Geometry: see drawing. Coordinates: mm, zero at the bounding-box minimum. A direction names the side the tool comes from. Round coordinates to 2 decimals unless told otherwise and drop trailing zeros. Order: outer loops, then holes, each group sorted by start corner. A loop starts at its lowest first (then second) coordinate and runs counter-clockwise, first axis right, second up. Notation, with made-up numbers: (-40, -7) - (-16, -7) arc R19 cw to (-16, 1) - close; hole circle Ø11 at (34, 36). An arc over 180 degrees is marked (long way). Put each result on its own line as item: value. Start each with the question number.
1) Line query: probe 1 along Y at (x, z) = (66.25, 0.65); probe 2 along Z at (x, y) = (16, 28.5); probe 3 along X at (y, z) = (20, 6.5). Output: solid intervals per line, ascending. Write a range as [from, to].
2) Section A-A on y = 28. Output: boundary loops of the cut face in (x, z), then the cut area to 3 significant figures.
3) Mould query, pull axis Y, two halves, no side actions, for the marked faces 1 and 2. Classes: +Y half, -Y half, draft (parallel to the pull), parting line (faces both ways), or undercut.
4) Section C-C on y = 11. Output: boundary loops of the cut face in (x, z).
5) Section D-D on z = 4.5. Output: boundary loops of the cut face in (x, y).
6) Contact query for flat-ended pins moving along their axis: P1, Ø5, axis at x = 57.5, y = 9.5, coming from the +Z side; P2, Ø5, axis at x = 66, y = 11, coming from the +Z side; P3, Ø0.8, axis at x = 65.5, z = 2.5, coming from the +Y side; P4, Ø4, axis at x = 10.5, z = 2.5, coming from the +Y side. Output: stop coordinate, or through.
7) Access query for the marked faces 3 and 4. Directions: +Z, -Z, +X, -X, +Y, -Y. A direction counts if a zero-diameter tool reaches every point of the face in a straight line with its end or side. Return the directions, or none.
8) Section B-B on x = 66.25. Output: boundary loops of the cut face in (y, z), then the cut area to 3 significant figures.
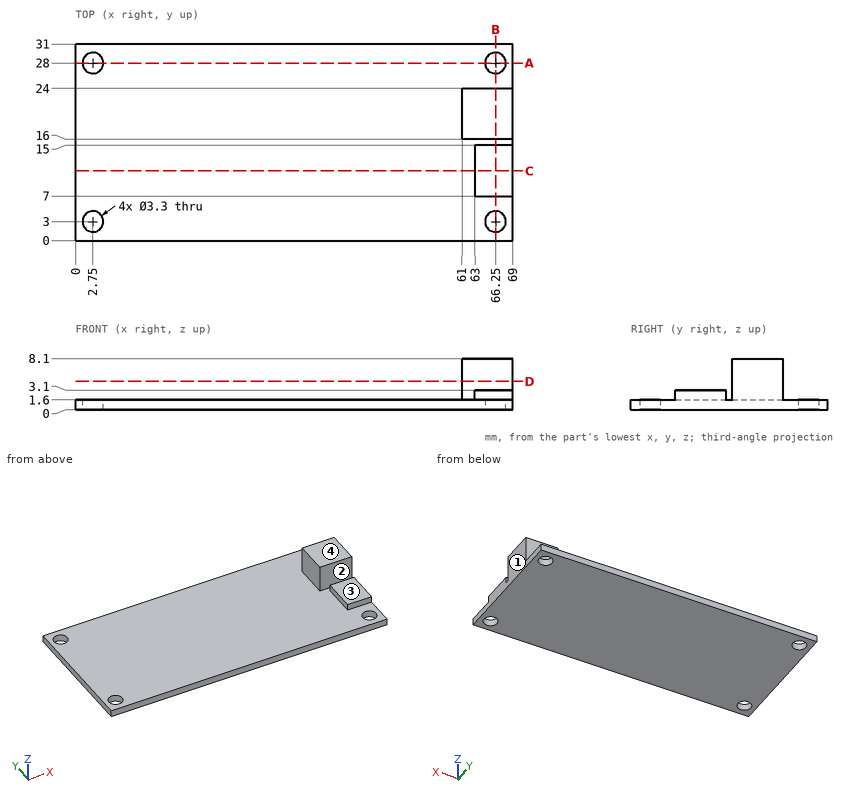
Answer sheet:
1. probe 1: [0, 1.35], [4.65, 26.35], [29.65, 31]
1. probe 2: [0, 1.6]
1. probe 3: [61, 69]
2. outline: (0, 0) - (1.1, 0) - (1.1, 1.6) - (0, 1.6) - close; (4.4, 0) - (64.6, 0) - (64.6, 1.6) - (4.4, 1.6) - close; (67.9, 0) - (69, 0) - (69, 1.6) - (67.9, 1.6) - close
2. area: 99.8 mm^2
3. face 1: draft
3. face 2: undercut
4. outline: (0, 0) - (69, 0) - (69, 3.1) - (63, 3.1) - (63, 1.6) - (0, 1.6) - close
5. outline: (61, 16) - (69, 16) - (69, 24) - (61, 24) - close
6. P1: z = 1.6
6. P2: z = 3.1
6. P3: y = 24
6. P4: y = 31
7. face 3: +Z, +X, -X, -Y
7. face 4: +Z, +X, -X, +Y, -Y
8. outline: (0, 0) - (1.35, 0) - (1.35, 1.6) - (0, 1.6) - close; (4.65, 0) - (26.35, 0) - (26.35, 1.6) - (24, 1.6) - (24, 8.1) - (16, 8.1) - (16, 1.6) - (15, 1.6) - (15, 3.1) - (7, 3.1) - (7, 1.6) - (4.65, 1.6) - close; (29.65, 0) - (31, 0) - (31, 1.6) - (29.65, 1.6) - close
8. area: 103 mm^2
